```python
from build123d import *

# Parameters (mm, degrees)
CROQUIS1_W              = 80
CROQUIS1_H              = 32
CROQUIS1_R              = 7.95
SALIENTE_EXTRUIR1_DEPTH = 13
CORTAR_EXTRUIR1_REACH   = 100.453
CROQUIS2_R              = 2.05
CROQUIS3_R              = 4
CORTAR_EXTRUIR2_DEPTH   = 5
REDONDEO1_R             = 10
CROQUIS4_W              = 5
CROQUIS4_H              = 16
SALIENTE_EXTRUIR2_DEPTH = 5
REDONDEO2_R             = 8


with BuildPart() as part:
    # Croquis1 → Saliente-Extruir1 (new body)
    with BuildSketch(Plane.XY):
        with Locations((30, -52)):
            Rectangle(CROQUIS1_W, CROQUIS1_H)
        with Locations(Location((53, -52, 0), (0, 0, 180))):
            Circle(CROQUIS1_R, mode=Mode.SUBTRACT)
    extrude(amount=SALIENTE_EXTRUIR1_DEPTH)

    # Croquis2 → Cortar-Extruir1 (cut, up to next)
    with BuildSketch(Plane.XY.offset(13), mode=Mode.PRIVATE) as cortar_extruir1_sk1:
        with Locations((0, -44)):
            Circle(CROQUIS2_R)
    cortar_extruir1_tool1 = extrude(cortar_extruir1_sk1.sketch, amount=-CORTAR_EXTRUIR1_REACH, mode=Mode.PRIVATE) & part.part
    # Croquis2 → Cortar-Extruir1 (cut, up to next)
    with BuildSketch(Plane.XY.offset(13), mode=Mode.PRIVATE) as cortar_extruir1_sk2:
        with Locations((20, -44)):
            Circle(CROQUIS2_R)
    cortar_extruir1_tool2 = extrude(cortar_extruir1_sk2.sketch, amount=-CORTAR_EXTRUIR1_REACH, mode=Mode.PRIVATE) & part.part
    # Croquis2 → Cortar-Extruir1 (cut, up to next)
    with BuildSketch(Plane.XY.offset(13), mode=Mode.PRIVATE) as cortar_extruir1_sk3:
        with Locations((0, -60)):
            Circle(CROQUIS2_R)
    cortar_extruir1_tool3 = extrude(cortar_extruir1_sk3.sketch, amount=-CORTAR_EXTRUIR1_REACH, mode=Mode.PRIVATE) & part.part
    # Croquis2 → Cortar-Extruir1 (cut, up to next)
    with BuildSketch(Plane.XY.offset(13), mode=Mode.PRIVATE) as cortar_extruir1_sk4:
        with Locations((20, -60)):
            Circle(CROQUIS2_R)
    cortar_extruir1_tool4 = extrude(cortar_extruir1_sk4.sketch, amount=-CORTAR_EXTRUIR1_REACH, mode=Mode.PRIVATE) & part.part
    add(cortar_extruir1_tool1.solids().sort_by_distance((0, -44, 13))[0], mode=Mode.SUBTRACT)
    add(cortar_extruir1_tool2.solids().sort_by_distance((20, -44, 13))[0], mode=Mode.SUBTRACT)
    add(cortar_extruir1_tool3.solids().sort_by_distance((0, -60, 13))[0], mode=Mode.SUBTRACT)
    add(cortar_extruir1_tool4.solids().sort_by_distance((20, -60, 13))[0], mode=Mode.SUBTRACT)

    # Croquis3 → Cortar-Extruir2 (cut)
    with BuildSketch(Plane.XY.offset(13)):
        with Locations((0, -44)):
            Circle(CROQUIS3_R)
        with Locations((20, -44)):
            Circle(CROQUIS3_R)
        with Locations((20, -60)):
            Circle(CROQUIS3_R)
        with Locations((0, -60)):
            Circle(CROQUIS3_R)
    extrude(amount=-CORTAR_EXTRUIR2_DEPTH, mode=Mode.SUBTRACT)

    # Redondeo1
    redondeo1_edges = [part.edges().sort_by_distance(p)[0] for p in [
        (70, -36, 6.5),
        (70, -68, 6.5),
    ]]
    fillet(redondeo1_edges, radius=REDONDEO1_R)

    # Croquis4 → Saliente-Extruir2 (add)
    with BuildSketch(Plane(origin=(0, 0, 0), x_dir=(-1, 0, 0), z_dir=(0, 0, -1))):
        with Locations((-32.5, -52)):
            Rectangle(CROQUIS4_W, CROQUIS4_H)
    extrude(amount=SALIENTE_EXTRUIR2_DEPTH)

    # Redondeo2
    # the kernel refuses this fillet: 8 mm, written as the material it adds along each edge
    with BuildSketch(Plane(origin=(35, -44, 0), x_dir=(1, 0, 0), z_dir=(0, -1, 0))) as redondeo2_piece_1:
        with BuildLine():
            CenterArc((7.416198487, -8), REDONDEO2_R, 90, 67.975687163)
            Line((0, -5), (-0.14832397, -4.94))
            ThreePointArc((-0.14832397, -4.94), (-0.16, -2.5), (-0.16, 0))
            Line((-0.16, 0), (0, 0.16))
            Line((0, 0.16), (7.416198487, 0.16))
            Line((7.416198487, 0.16), (7.416198487, 0))
        make_face()
    extrude(amount=16)


solid = part.part
```
Input: part model. Units: mm. Frame: model coordinates. A direction names the side the tool comes from. Coordinates: 2 decimals unless noted, no trailing zeros. Loops run counter-clockwise (first coordinate to the right, second up) from the corner with the lowest first, then second, coordinate; pieces in that order, holes last.
Q1. Contact query for flat-ended pins moving along their axis: pin 1 (6.5 mm diameter, centred on x = 20, y = -60, fed in from +Z); pin 2 (12 mm diameter, centred on x = 2, y = -56, fed in from -Z); pin 3 (9.5 mm diameter, centred on x = 28.5, y = -51, fed in from -Z); pin 4 (1 mm diameter, centred on y = -44.5, z = -1, fed in from -X). Output: stop coordinate, or through.
Results are:
pin 1: stops at z = 8
pin 2: stops at z = 0
pin 3: stops at z = -5
pin 4: stops at x = 30
Q2. Section B-B, the plane x = 53. Return the cut outline in (y, z), and give its area (3 significant figures).
Results are:
outline: (-68, 0) - (-59.95, 0) - (-59.95, 13) - (-68, 13) - close; (-44.05, 0) - (-36, 0) - (-36, 13) - (-44.05, 13) - close
area: 209 mm2
Q3. Line query: line 1 along Y through (x, z) = (0, 2.5); line 2 along Y through (x, z) = (20, 9.3); line 3 along Y through (x, z) = (53, 8.25). Output: solid intervals per line, ascending.
Results are:
line 1: y = -68 to -62.05, -57.95 to -46.05, -41.95 to -36
line 2: y = -68 to -64, -56 to -48, -40 to -36
line 3: y = -68 to -59.95, -44.05 to -36
Q4. Section A-A, the plane x = 20. Return the cut outline in (y, z).
Results are:
outline: (-68, 0) - (-62.05, 0) - (-62.05, 8) - (-64, 8) - (-64, 13) - (-68, 13) - close; (-57.95, 0) - (-46.05, 0) - (-46.05, 8) - (-48, 8) - (-48, 13) - (-56, 13) - (-56, 8) - (-57.95, 8) - close; (-41.95, 0) - (-36, 0) - (-36, 13) - (-40, 13) - (-40, 8) - (-41.95, 8) - close
Q5. Set-up query: faces 1 (the flat face through (34, -44, -2)), 2 (the cylindrical face through (48.726, -58.703, 6.409)), 3 (the cylindrical face through (38, -51.89, -1.33)), 4 (the flat face through (30, -52, -2)), 5 (the cylindrical face through (-0.867, -63.905, 10.535)). Return all of +Z, -Z, +X, -X, +Y, -Y with unobstructed straight access to the full face (end or side cutting, diameter ignored); none if empty.
Results are:
face 1: -Z, +X, -X, +Y
face 2: +Z, -Z
face 3: -Z, +X, +Y, -Y
face 4: -Z, -X, +Y, -Y
face 5: +Z
Q6. Section D-D, the plane z = 2.25. Return the cut outline in (x, y), and give its area (3 significant figures).
Results are:
outline: (-10, -68) - (60, -68) arc R10 ccw to (70, -58) - (70, -46) arc R10 ccw to (60, -36) - (-10, -36) - close; hole circle Ø4.1 at (0, -60); hole circle Ø4.1 at (0, -44); hole circle Ø4.1 at (20, -60); hole circle Ø4.1 at (20, -44); hole circle Ø15.9 at (53, -52)
area: 2,270 mm2
Q7. Mould query, pull axis Y, two halves, no side actions, for faces 6 (the flat face through (25, -36, 6)), 7 (the cylindrical face through (-0.267, -57.967, 4.056)), 8 (the flat face through (25, -68, 6)). Classes: +Y half, -Y half, draft (parallel to the pull), parting line (faces both ways), or undercut.
Results are:
face 6: +Y half
face 7: undercut
face 8: -Y half
Q8. Section C-C, the plane y = -50. Return the cut outline in (x, z).
Results are:
outline: (-10, 0) - (30, 0) - (30, -5) - (35, -5) arc R8 cw to (42.42, 0) - (45.31, 0) - (45.31, 13) - (-10, 13) - close; (60.69, 0) - (70, 0) - (70, 13) - (60.69, 13) - close
